```python
from build123d import *

# Parameters (mm, degrees)
SKETCH_R              = 66
PAD_DEPTH             = 15
SKETCH001_R           = 32
POCKET_DEPTH          = 389.556737
POLARPATTERN_COUNT    = 8
POCKET001_DEPTH       = 378.893286
POLARPATTERN001_COUNT = 8
PAD001_DEPTH          = 10
SKETCH004_R           = 18
PAD002_DEPTH          = 3
SKETCH005_R           = 18
PAD003_DEPTH          = 3
SKETCH006_R           = 8
POCKET002_DEPTH       = 31.001
SKETCH007_R           = 15
PAD004_DEPTH          = 18
SKETCH008_R           = 8
PAD005_DEPTH          = 31
SKETCH009_R           = 4
PAD006_DEPTH          = 3
SKETCH010_R           = 5
PAD007_DEPTH          = 10
FILLET_R              = 2
FILLET001_R           = 2


with BuildPart() as part:
    # Sketch → Pad (new body)
    with BuildSketch(Plane.YZ):
        Circle(SKETCH_R)
    extrude(amount=PAD_DEPTH)

    # Sketch001 (on Face3 of Pad) → Pocket (cut, through all)
    with BuildSketch(Plane.YZ.offset(15)):
        with Locations((-92, 0)):
            Circle(SKETCH001_R)
    pocket = extrude(amount=-POCKET_DEPTH, mode=Mode.SUBTRACT)

    # PolarPattern: Pocket ×8 about axis
    polarpattern_axis = Axis((15, 0, 0), (1, 0, 0))
    for i in range(1, POLARPATTERN_COUNT):
        add(pocket.rotate(polarpattern_axis, i * 360 / POLARPATTERN_COUNT), mode=Mode.SUBTRACT)

    # Sketch002 (on Face1 of PolarPattern) → Pocket001 (cut, through all)
    with BuildSketch(Plane.YZ.offset(15)):
        with BuildLine():
            ThreePointArc((-63.774583, 30.745866), (-69.000835, 28.581082), (-66.836051, 23.35483))
            Line((-66.836051, 23.35483), (-42.181433, 13.142553))
            ThreePointArc((-42.181433, 13.142553), (-36.955181, 15.307337), (-39.119966, 20.533589))
            Line((-39.119966, 20.533589), (-63.774583, 30.745866))
        make_face()
    pocket001 = extrude(amount=-POCKET001_DEPTH, mode=Mode.SUBTRACT)

    # PolarPattern001: Pocket001 ×8 about axis
    polarpattern001_axis = Axis((15, 0, 0), (1, 0, 0))
    for i in range(1, POLARPATTERN001_COUNT):
        add(pocket001.rotate(polarpattern001_axis, i * 360 / POLARPATTERN001_COUNT), mode=Mode.SUBTRACT)

    # Sketch003 (on Face1 of PolarPattern001) → Pad001 (join)
    with BuildSketch(Plane.YZ.offset(15)):
        with BuildLine():
            ThreePointArc((9.42809, 33.333333), (0, 40), (-9.42809, 33.333333))
            Line((-9.42809, 33.333333), (-18.856181, 6.666667))
            ThreePointArc((-18.856181, 6.666667), (0, -20), (18.856181, 6.666667))
            Line((18.856181, 6.666667), (9.42809, 33.333333))
        make_face()
    extrude(amount=PAD001_DEPTH)

    # Sketch004 (on Face55 of Pad001) → Pad002 (join)
    with BuildSketch(Plane.YZ.offset(25)):
        Circle(SKETCH004_R)
    extrude(amount=PAD002_DEPTH)

    # Sketch005 (on Face54 of Pad002) → Pad003 (join)
    with BuildSketch(Plane(origin=(0, 0, 0), x_dir=(0, 1, 0), z_dir=(-1, 0, 0))):
        Circle(SKETCH005_R)
    extrude(amount=PAD003_DEPTH)

    # Sketch006 (on Face59 of Pad003) → Pocket002 (cut, through all)
    with BuildSketch(Plane.YZ.offset(28)):
        Circle(SKETCH006_R)
    extrude(amount=-POCKET002_DEPTH, mode=Mode.SUBTRACT)

    # Sketch007 (on Face58 of Pocket002) → Pad004 (join)
    with BuildSketch(Plane(origin=(-3, 0, 0), x_dir=(0, 1, 0), z_dir=(-1, 0, 0))):
        Circle(SKETCH007_R)
    extrude(amount=PAD004_DEPTH)

    # Sketch008 (on Face62 of Pad004) → Pad005 (join)
    with BuildSketch(Plane(origin=(-21, 0, 0), x_dir=(0, 1, 0), z_dir=(-1, 0, 0))):
        Circle(SKETCH008_R)
    extrude(amount=PAD005_DEPTH)

    # Sketch009 (on Face65 of Pad005) → Pad006 (join)
    with BuildSketch(Plane(origin=(-52, 0, 0), x_dir=(0, 1, 0), z_dir=(-1, 0, 0))):
        Circle(SKETCH009_R)
    extrude(amount=PAD006_DEPTH)

    # Sketch010 (on Face67 of Pad006) → Pad007 (join)
    with BuildSketch(Plane(origin=(-55, 0, 0), x_dir=(0, 1, 0), z_dir=(-1, 0, 0))):
        Circle(SKETCH010_R)
    extrude(amount=PAD007_DEPTH)

    # Fillet
    fillet_edges = [part.edges().sort_by_distance(p)[0] for p in [
        (0, -18, 0),
    ]]
    fillet(fillet_edges, radius=FILLET_R)

    # Fillet001
    fillet001_edges = [part.edges().sort_by_distance(p)[0] for p in [
        (15, 0, -20),
    ]]
    fillet(fillet001_edges, radius=FILLET001_R)


solid = part.part
```
Geometry check sheet. Reference: the model listing, model coordinates, mm. A direction names the side the tool comes from. Give positions to 0.01 mm unless a question says otherwise; leave off trailing zeros. Order: outer loops, then holes, each group sorted by start corner. A loop starts at its lowest first (then second) coordinate and runs counter-clockwise, first axis right, second up. Notation, with made-up numbers: (-14.5, 33.5) - (43.5, 33.5) arc R22 ccw to (43.5, 56.5) - close; hole circle Ø10 at (78, 87.25). An arc over 180 degrees is marked (long way). Answer in a Markdown table with one row per item. Add a question column.
Q1. Mould release check, pull along Y, two halves, no side actions. Record for faces 4 (the flat face through (7.6, 24.78, -49.37)), 5 (the cylindrical face through (21, 0, 40)), 6 (the cylindrical face through (8, -60, 0)), 7 (the cylindrical face through (7.4, 18.58, -63.33)): pulls with the +Y half, pulls with the -Y half, needs draft (parallel to the pull), parting line crosses it, or undercut.
Q2. Tool access check on faces 1 (the flat face through (7.6, -17.27, 52.15)), 2 (the cylindrical face through (26.479, -2.343, 17.847)), 3 (the flat face through (-3, -4, -15)). Record the directions out of +Z, -Z, +X, -X, +Y, -Y that give a thin tool (end or side, any length) a straight path to the whole face; none if there is none.
Q3. Cross-section at B-B, the plane x = -41.5. Enter the section's corners in (y, z), then the cut area to 3 significant figures.
Q4. Gauge pin test, flat ends, axial feed: pin 1 (8 mm diameter, centred on y = 1.5, z = -1.5, fed in from +X); pin 2 (12 mm diameter, centred on y = -17.5, z = -23, fed in from +X); pin 3 (12 mm diameter, centred on x = 14.5, z = -2, fed in from +Y). Record the tip position at first contact, or that the pin passes through.
Q5. Cross-section at C-C, the plane z = -27. Enter the section's corners in (x, y), then the cut area to 3 significant figures.
Q6. Cross-section at A-A, the plane z = -47.5. Enter the section's corners in (x, y).
Q7. Material ranges on probe 1 along Z at (x, y) = (4, 0); probe 2 along Z at (x, y) = (17.5, 0); probe 3 along X at (y, z) = (45, 39), recorded low to high. Write a range as from..to.
Check values:
| question | item | result |
|---|---|---|
| 1 | face 4 | undercut |
| 1 | face 5 | parting line crosses it |
| 1 | face 6 | pulls with the -Y half |
| 1 | face 7 | pulls with the +Y half |
| 2 | face 1 | +X, -X |
| 2 | face 2 | +X |
| 2 | face 3 | -X |
| 3 | outline | circle Ø16 at (0, 0) |
| 3 | area | 201 mm^2 |
| 4 | pin 1 | stops at x = -3 |
| 4 | pin 2 | stops at x = 15 |
| 4 | pin 3 | stops at y = 61.02 |
| 5 | outline | (0, -54.73) - (15, -54.73) - (15, 54.73) - (0, 54.73) - close |
| 5 | area | 1,640 mm^2 |
| 6 | outline | (0, -38.3) - (15, -38.3) - (15, -24) - (0, -24) - close; (0, -15.35) - (15, -15.35) - (15, 15.35) - (0, 15.35) - close; (0, 24) - (15, 24) - (15, 38.3) - (0, 38.3) - close |
| 7 | probe 1 | z = -60..-8, 8..60 |
| 7 | probe 2 | z = -20..-8, 8..40 |
| 7 | probe 3 | x = 0..15 |
